Drawing for the job (mm, zero at the part's lowest x, y, z). A direction names the side the tool comes from. Round coordinates to 2 decimals unless told otherwise and drop trailing zeros. Order: outer loops, then holes, each group sorted by start corner. A loop starts at its lowest first (then second) coordinate and runs counter-clockwise, first axis right, second up. Notation, with made-up numbers: (14.5, 47) - (55.5, 47) arc R22 cw to (55.5, 74) - close; hole circle Ø5 at (-32, 51.5). An arc over 180 degrees is marked (long way). One line per question, with ' | ' between items. Start each with the question number.
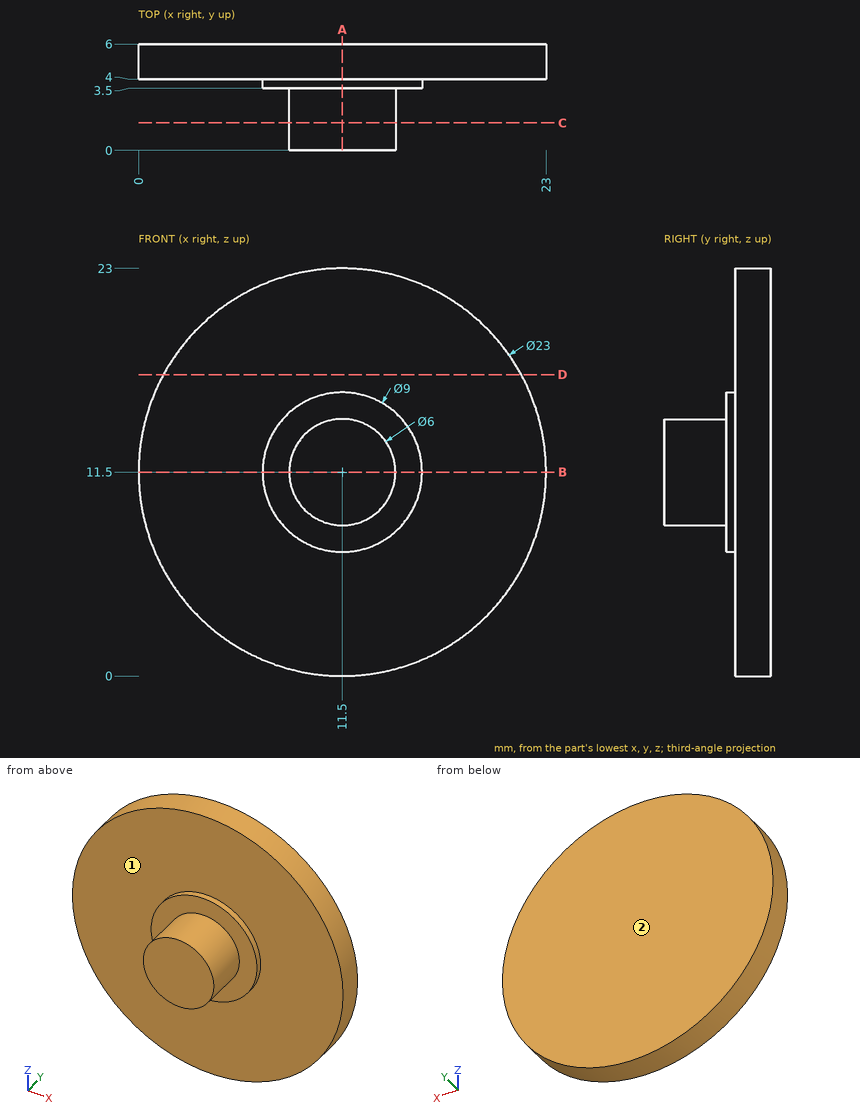
Item 1: Pin check, flat tips, straight feed: pin 1 (3 mm diameter, centred on x = 12.5, y = 1.5, fed in from -Z); pin 2 (2 mm diameter, centred on x = 8, y = 5.5, fed in from +Z) (3 decimals); pin 3 (7 mm diameter, centred on x = 12.5, z = 15.5, fed in from -Y); pin 4 (1 mm diameter, centred on y = 4, z = 10.5, fed in from +X). Stop position of each tip, or through.
Item 2: Slice it at A-A (x = 11.5). Write the cut outline in (y, z), plus the area to 3 significant figures.
Item 3: Slice it at C-C (y = 1.55). Write the cut outline in (x, z), plus the area to 3 significant figures.
Item 4: 3-axis set-ups, long thin cutter, end or side, ignore diameter. For the marked faces 1 and 2: which of +Z, -Z, +X, -X, +Y, -Y reach the whole face in a straight line?
Item 5: Slice it at B-B (z = 11.5). Write the cut outline in (x, y), plus the area to 3 significant figures.
Item 6: Wall check: line 1 along Y through (x, z) = (7.75, 14.5); line 2 along Y through (x, z) = (12.25, 15.75); line 3 along X through (y, z) = (2.45, 10.75). Give the ranges that are in metal, low to high. Write a range as [from, to].
Item 7: Slice it at D-D (z = 17). Write the cut outline in (x, y).
A:
1) pin 1: z = 8.5 | pin 2: z = 22.725 | pin 3: y = 0 | pin 4: x = 22.99
2) outline: (0, 8.5) - (3.5, 8.5) - (3.5, 7) - (4, 7) - (4, 0) - (6, 0) - (6, 23) - (4, 23) - (4, 16) - (3.5, 16) - (3.5, 14.5) - (0, 14.5) - close | area: 71.5 mm^2
3) outline: circle Ø6 at (11.5, 11.5) | area: 28.3 mm^2
4) face 1: -Y | face 2: +Z, -Z, +X, -X, +Y
5) outline: (0, 4) - (7, 4) - (7, 3.5) - (8.5, 3.5) - (8.5, 0) - (14.5, 0) - (14.5, 3.5) - (16, 3.5) - (16, 4) - (23, 4) - (23, 6) - (0, 6) - close | area: 71.5 mm^2
6) line 1: [4, 6] | line 2: [3.5, 6] | line 3: [8.6, 14.4]
7) outline: (1.4, 4) - (21.6, 4) - (21.6, 6) - (1.4, 6) - close
